Read the model definition and answer for the solid it produces. Units are mm, in the model's axes. Face numbers are marked on the shaded views. Coordinates: 2 decimals unless noted, no trailing zeros. Loops run counter-clockwise (first coordinate to the right, second up) from the corner with the lowest first, then second, coordinate; pieces in that order, holes last. Notation, with made-up numbers: (29, -8.5) - (66, -8.5) arc R12 ccw to (66, 9.5) - close; hole circle Ø1 at (87, 57.25). An arc over 180 degrees is marked (long way). Use one line per item in the form item = value. Start each with the question number.
1) A cutting plane is placed at A-A (z = 100). Give the vertices of the cut face in (x, y).
2) Consider line 1 (Z direction, x = 54.5, y = -3); line 2 (X direction, y = -19, z = 100); line 3 (X direction, y = -13, z = 138). Determine where each line is inside the solid, lowest interval first.
3) A cutting plane is placed at D-D (x = 75.5). Give the vertices of the cut face in (y, z), and give its area (3 significant figures).
4) The mould has two halves that part along Z. Classify the marked faces 1, 2, 3 and 4: released by +Z, released by -Z, zero draft, split by the parting line, or undercut.
5) Each of these flat-tipped pins is pushed along its axis until it touches: P1, Ø10, axis at y = -7.5, z = 148, coming from the +X side (3 decimals); P2, Ø6, axis at x = 63, y = -10.5, coming from the +Z side. Where does it stop, or does it pass through?
6) A cutting plane is placed at B-B (x = -24). Give the vertices of the cut face in (y, z), and give its area (3 significant figures).
7) A cutting plane is placed at C-C (y = -26.5). Give the vertices of the cut face in (x, z) (3 decimals).
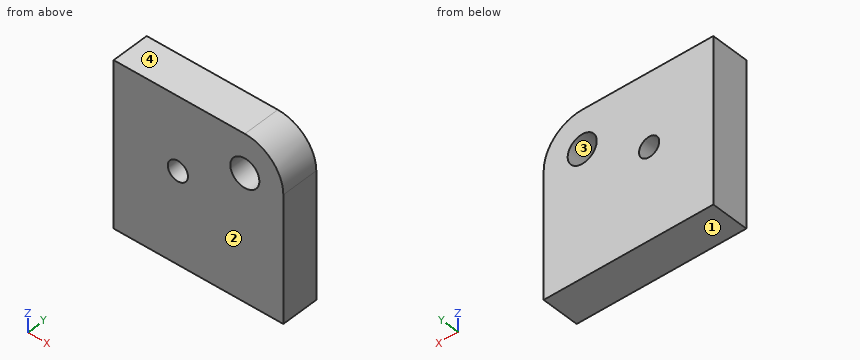
Autodesk Inventor part; units mm, degrees
ref_plane "YZ Plane" through (0, 0, 0) normal (1, 0, 0) x (0, 1, 0)
ref_plane "XZ Plane" through (0, 0, 0) normal (0, 1, 0) x (-1, 0, 0)
ref_plane "XY Plane" through (0, 0, 0) normal (0, 0, 1) x (1, 0, 0)
sketch "Эскиз1" plane through (0, 0, 0) normal (0, 0, 1) x (1, 0, 0)
  line L0 (-88.1763, -30) -> (96.8237, -30)
  line L1 (-88.1763, -30) -> (-88.1763, 11)
  line L2 (96.8237, 11) -> (96.8237, -30)
  line L3 (-88.1763, 11) -> (96.8237, 11)
  point P0 (0, 0)
  point P1 (0, -30)
  dimension "parametr_A" = 185
  dimension "parametr_C" = 41
extrude "Выдавливание2" add sketch "Эскиз1" along normal blind 180
fillet "Сопряжение1" radius 42 1 edges at (96.8237, -9.5, 180)
sketch "Эскиз5" plane through (-88.1763, -30, 0) normal (0, -1, 0) x (1, 0, 0)
  point P0 (70, 100)
hole "Отверстие5" at (-18.1763, -30, 100) direction (0, 1, 0) diameter 22 end through all
sketch "Эскиз7" plane through (-88.1763, 11, 0) normal (0, 1, 0) x (1, 0, 0)
  point P0 (143, -138)
hole "Отверстие7" at (54.8237, 11, 138) direction (0, -1, 0) diameter 31.67 depth 96 tip angle 120
sketch "Эскиз2" plane through (-88.1763, -30, 0) normal (0, -1, 0) x (1, 0, 0)
  point P0 (114.3354, 27.5417)
sketch "Эскиз3" plane through (-88.1763, -30, 0) normal (0, -1, 0) x (1, 0, 0)
  point P0 (14.3354, 15.8973)
equation "\"parametr_A\" = parametr_A_"
equation "\"parametr_C\" = parametr_D_"
equation "\"paramert_B\" = parametr_B_"
equation "\"d21\" = parametr_G_"
equation "\"parametr_A_\" = 185"
equation "\"parametr_B_\" = 180"
equation "\"parametr_D_\" = 41"
equation "\"parametr_E_\" = 35"
equation "\"parametr_G_\" = 42"
properties part number "lw_6_part1"
Found:
q1.outline = (-88.18, -30) - (-29.18, -30) - (-29.18, 11) - (-88.18, 11) - close; (-7.18, -30) - (96.82, -30) - (96.82, 11) - (-7.18, 11) - close
q2.line_1 = 0 to 122.17, 153.83 to 180
q2.line_2 = -88.18 to -29.18, -7.18 to 96.82
q2.line_3 = -88.18 to 38.99, 70.66 to 96.82
q3.outline = (-30, 0) - (11, 0) - (11, 174.56) - (-30, 174.56) - close
q3.area = 7,160 mm^2
q4.face_1 = released by -Z
q4.face_2 = zero draft
q4.face_3 = undercut
q4.face_4 = released by +Z
q5.P1 = 96.525
q5.P2 = 179.68
q6.outline = (-30, 0) - (11, 0) - (11, 90.67) - (-30, 90.67) - close; (-30, 109.33) - (11, 109.33) - (11, 180) - (-30, 180) - close
q6.area = 6,610 mm^2
q7.outline = (-88.176, 0) - (96.824, 0) - (96.824, 138) arc R42 ccw to (54.824, 180) - (-88.176, 180) - close; hole circle Ø22 at (-18.176, 100); hole circle Ø31.67 at (54.824, 138)
